```python
from build123d import *

# Parameters (mm, degrees)
SKETCH_1_R      = 3.35
EXTRUDE_1_DEPTH = 20


with BuildPart() as part:
    # 草图1 → 凸台-拉伸1 (new body)
    with BuildSketch(Plane(origin=(0, 0, 0), x_dir=(1, 0, 0), z_dir=(0, 1, 0))):
        with BuildLine():
            Line((-5.997922074, -0.157894881), (-2.104603424, -148.052632133))
            ThreePointArc((-2.104603424, -148.052632133), (-0.106718985, -150), (1.893934378, -148.055476932))
            Line((1.893934378, -148.055476932), (5.99769133, -0.166429278))
            ThreePointArc((5.99769133, -0.166429278), (0.004268758, 5.999998481), (-5.997922074, -0.157894881))
        make_face()
        with Locations(Location((0, 0, 0), (0, 0, 270))):
            Circle(SKETCH_1_R, mode=Mode.SUBTRACT)
    extrude(amount=EXTRUDE_1_DEPTH)


solid = part.part
```
Here's how the part is built. I have some questions about the finished solid (model axes, mm). Round coordinates to 2 decimals unless told otherwise and drop trailing zeros. Write each loop counter-clockwise with the first axis right and the second up, starting at its lowest first coordinate (ties: lowest second). Pieces come first, ordered by that corner, then holes.
Q1. If we section it at B-B on y = 13: Write out the boundary of the cut face in (x, z).
Q2. If we section it at A-A on x = 0: Write out the boundary of the cut face in (y, z), plus the area to 3 significant figures.
Q3. Will these pins go through, and if not, where does the flat tip stop? P1, Ø1, axis at x = -4.5, z = 30, coming from the -Y side; P2, Ø1.5, axis at y = 14.5, z = 99.5, coming from the -X side; P3, Ø6, axis at x = -4, y = 6.5, coming from the -Z side; P4, Ø5, axis at y = 10.5, z = 81, coming from the -X side.
Q4. If we section it at C-C on z = 117: Write out the boundary of the cut face in (x, y), plus the area to 3 significant figures.
Q5. If we mould it in two halves opening along X, with no side actions, what happens to faces 1 (the flat face through (0, 0, 71)), 2 (the cylindrical face through (-2.038, 9.86, -2.658)), 3 (the cylindrical face through (-0.1, 9.9, 150))? For each: +X half, -X half, draft (parallel to the pull), parting line (faces both ways), or undercut.
Q6. Please list where these lines run through material, in increasing order: probe 1 along X at (y, z) = (14.25, 0); probe 2 along Z at (x, y) = (-0.25, 18.5); probe 3 along Z at (x, y) = (-1.5, 11).
Answer below:
1. outline: (-6, 0.16) arc R6 ccw (long way) to (6, 0.17) - (1.89, 148.06) arc R2 ccw to (-2.1, 148.05) - close; hole circle Ø6.7 at (0, 0)
2. outline: (0, -6) - (20, -6) - (20, -3.35) - (0, -3.35) - close; (0, 3.35) - (20, 3.35) - (20, 150) - (0, 150) - close
2. area: 2,990 mm2
3. P1: stops at y = 0
3. P2: stops at x = -3.4
3. P3: stops at z = -5.92
3. P4: stops at x = -3.94
4. outline: (-2.92, 0) - (2.76, 0) - (2.76, 20) - (-2.92, 20) - close
4. area: 114 mm2
5. face 1: draft
5. face 2: undercut
5. face 3: parting line
6. probe 1: x = -6 to -3.35, 3.35 to 6
6. probe 2: z = -5.99 to -3.34, 3.34 to 149.99
6. probe 3: z = -5.81 to -3, 3 to 149.43
